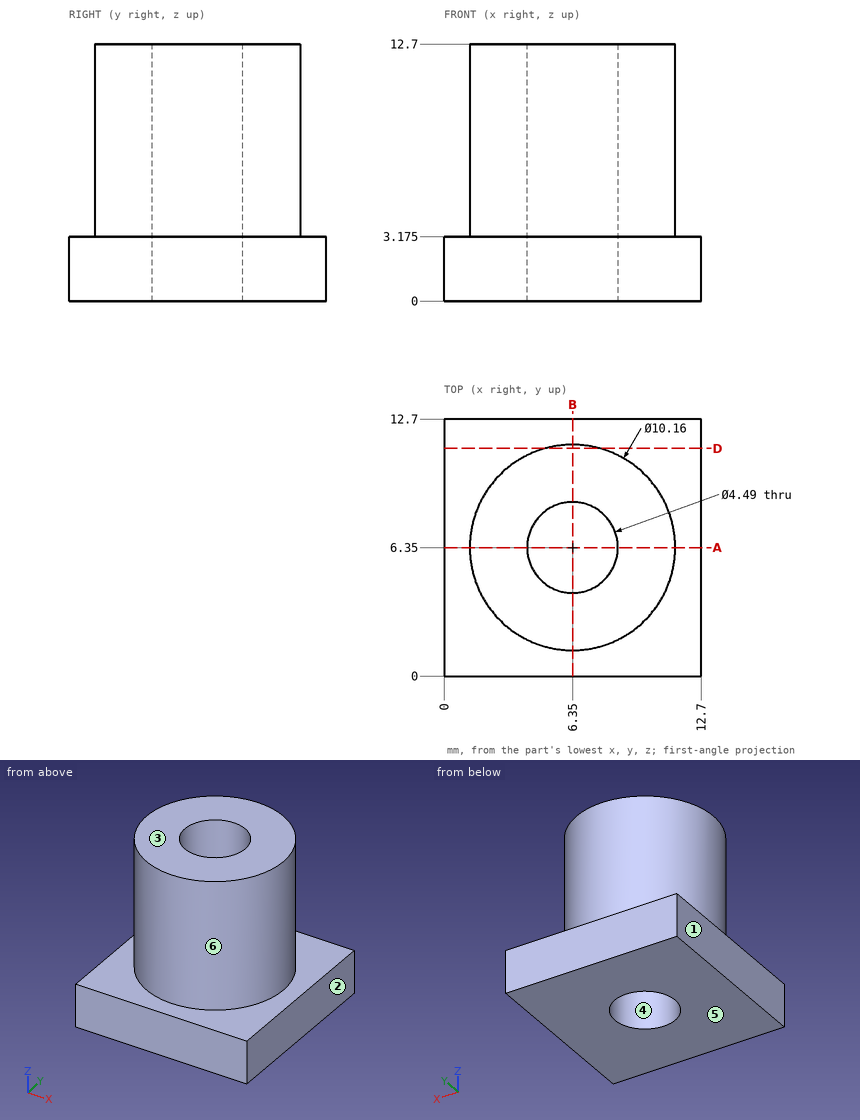
Answer from the drawing. Dimensions are ordinates in mm from the lowest x, y and z of the part. A direction names the side the tool comes from. Round coordinates to 2 decimals unless told otherwise and drop trailing zeros. Write each loop counter-clockwise with the first axis right and the second up, starting at its lowest first coordinate (ties: lowest second). Pieces come first, ordered by that corner, then holes. Notation, with made-up numbers: (55.5, -9.5) -> (84.5, -9.5) arc R21 ccw to (84.5, 7.5) -> close; hole circle Ø9 at (-3, 39). An arc over 180 degrees is marked (long way). Answer in a Markdown table with one row per item. Add a question column.
1) Find section A-A, the plane y = 6.35. Determine the outline of the cut face in (x, z) (1 decimal).
2) Given P1, Ø1, axis at y = 2.5, z = 6.5, coming from the +X side; P2, Ø3, axis at x = 7.5, z = 8.5, coming from the -Y side, each flat-ended and moving along its own axis, determine where each tip first touches the part or whether it passes through.
3) Determine the mould class of the marked faces 1, 2, 3 and 4 for opening direction X: pulls with the +X half, pulls with the -X half, needs draft (parallel to the pull), parting line crosses it, or undercut.
4) Consider line 1 (Y direction, x = 6.35, z = 7.5) (1 decimal); line 2 (Z direction, x = 1.75, y = 2.75) (3 decimals); line 3 (X direction, y = 4.5, z = 9). Determine where each line is inside the solid, lowest interval first.
5) Which of the six approach directions +Z, -Z, +X, -X, +Y, -Y give full straight-line access (tool end or side, diameter ignored) to the marked faces 5 and 6?
6) Find section D-D, the plane y = 11.25. Determine the outline of the cut face in (x, z) (1 decimal).
Findings below:
| question | item | result |
|---|---|---|
| 1 | outline | (0, 0) -> (4.1, 0) -> (4.1, 12.7) -> (1.3, 12.7) -> (1.3, 3.2) -> (0, 3.2) -> close; (8.6, 0) -> (12.7, 0) -> (12.7, 3.2) -> (11.4, 3.2) -> (11.4, 12.7) -> (8.6, 12.7) -> close |
| 2 | P1 | x = 10.17 |
| 2 | P2 | y = 1.27 |
| 3 | face 1 | pulls with the -X half |
| 3 | face 2 | pulls with the +X half |
| 3 | face 3 | needs draft |
| 3 | face 4 | undercut |
| 4 | line 1 | 1.3 to 4.1, 8.6 to 11.4 |
| 4 | line 2 | 0 to 3.175 |
| 4 | line 3 | 1.62 to 5.08, 7.62 to 11.08 |
| 5 | face 5 | -Z, +X, -X, +Y, -Y |
| 5 | face 6 | +Z |
| 6 | outline | (0, 0) -> (12.7, 0) -> (12.7, 3.2) -> (7.7, 3.2) -> (7.7, 12.7) -> (5, 12.7) -> (5, 3.2) -> (0, 3.2) -> close |
